Input: part model. Units: mm. Frame: model coordinates. Face numbers are marked on the shaded views. A direction names the side the tool comes from. Give positions to 0.01 mm unless a question says otherwise; leave off trailing zeros. Order: outer loops, then holes, each group sorted by start corner. A loop starts at its lowest first (then second) coordinate and runs counter-clockwise, first axis right, second up. Notation, with made-up numbers: (89, 17.25) - (110, 17.25) arc R31 ccw to (110, 42.25) - close; hole circle Ø6 at (46, -7). An arc over 180 degrees is marked (long way). Answer in a Markdown table with one row per item. Add a question column.
1. Ray query, line 1 (X direction, y = -9.5, z = -8); line 2 (Y direction, x = -27, z = -0.25); line 3 (Y direction, x = -21.5, z = -0.75). Return the intervals inside material, ascending. Write a range as [from, to].
2. Section query C-C on x = -14. Return loops of the section in (y, z).
3. Access query for the marked faces 1 and 2. Directions: +Z, -Z, +X, -X, +Y, -Y. A direction counts if a zero-diameter tool reaches every point of the face in a straight line with its end or side. Return the directions, or none.
4. Mould query, pull axis X, two halves, no side actions, for the marked faces 3, 4 and 5. Classes: released by +X, released by -X, zero draft, split by the parting line, or undercut.
5. Section query D-D on y = -22.5. Return loops of the section in (x, z).
6. Section query A-A on y = -14. Return loops of the section in (x, z).
7. Section query B-B on z = -0.5. Count the separate pieces of the cut face and the enclosed holes in it, and give its area (3 significant figures).
8. Contact query for flat-ended pins moving along their axis: pin 1 (1.2 mm diameter, centred on x = -14, y = -29, fed in from -Z); pin 2 (1.9 mm diameter, centred on x = -20, y = -2.5, fed in from -Z); pin 3 (0.5 mm diameter, centred on y = -29.5, z = -9, fed in from -X). Output: stop coordinate, or through.
```python
from build123d import *

# Parameters (mm, degrees)
SKETCH_2_W          = 31.092354585
SKETCH_2_H          = 31.600355601
EXTRUDE_1_DEPTH     = 1.5
SKETCH_3_R          = 1.9
SKETCH_3_R_2        = 0.85
EXTRUDE_2_DEPTH     = 2
SKETCH_4_W          = 31.092354585
SKETCH_4_H          = 31.600355601
SKETCH_4_R          = 0.9
SKETCH_4_R_2        = 0.95
EXTRUDE_3_DEPTH     = 13
CUT_EXTRUDE_1_REACH = 46.929
SKETCH_5_R          = 0.5
SKETCH_5_W          = 3.540807658
SKETCH_5_H          = 9.178364527
CUT_EXTRUDE_2_REACH = 46.95
SKETCH_6_W          = 4.41346869
SKETCH_6_H          = 8.209522231
CUT_EXTRUDE_3_REACH = 46.95
SKETCH_8_W          = 1
SKETCH_8_H          = 4
FILLET_1_R          = 1
FILLET_2_R          = 0.8


with BuildPart() as part:
    # 草图2 → 凸台-拉伸1 (new body)
    with BuildSketch(Plane.XY):
        with Locations((-13.658877318, -13.912877826)):
            Rectangle(SKETCH_2_W, SKETCH_2_H)
    extrude(amount=EXTRUDE_1_DEPTH)

    # 草图3 → 凸台-拉伸2 (add)
    # profile 1 of 2: a face of its own
    with BuildSketch(Plane(origin=(0, 0, 0), x_dir=(-1, 0, 0), z_dir=(0, 0, -1))):
        with Locations(Location((20.20004064, -2.16000508, 0), (0, 0, 180))):
            Circle(SKETCH_3_R)
        with Locations(Location((20.20004064, -2.16000508, 0), (0, 0, 180))):
            Circle(SKETCH_3_R_2, mode=Mode.SUBTRACT)
    # profile 2 of 2: a face of its own
    with BuildSketch(Plane(origin=(0, 0, 0), x_dir=(-1, 0, 0), z_dir=(0, 0, -1))):
        with Locations(Location((7.24001524, -25.6500508, 0), (0, 0, 180))):
            Circle(SKETCH_3_R)
        with Locations(Location((7.24001524, -25.6500508, 0), (0, 0, 180))):
            Circle(SKETCH_3_R_2, mode=Mode.SUBTRACT)
    extrude(amount=EXTRUDE_2_DEPTH)

    # 草图4 → 凸台-拉伸3 (add)
    # profile 1 of 2: a face of its own
    with BuildSketch(Plane(origin=(0, 0, 0), x_dir=(-1, 0, 0), z_dir=(0, 0, -1))):
        with Locations((13.658877318, -13.912877826)):
            Rectangle(SKETCH_4_W, SKETCH_4_H)
        Polygon((-0.387299975, -28.213055626), (-0.387299975, -23.216633759), (-0.387299975, 0.387299975), (22.708632743, 0.387299975), (27.70505461, 0.387299975), (27.70505461, -28.213055626), align=None, mode=Mode.SUBTRACT)
    # profile 2 of 2: a face of its own
    with BuildSketch(Plane(origin=(0, 0, 0), x_dir=(-1, 0, 0), z_dir=(0, 0, -1))):
        with BuildLine():
            Line((22.708632743, -28.200355601), (4.596421868, -28.200355601))
            ThreePointArc((4.596421868, -28.200355601), (3.261678652, -24.551376974), (-0.387299975, -23.216633759))
            Line((-0.387299975, -23.216633759), (-0.387299975, -28.213055626))
            Line((-0.387299975, -28.213055626), (27.70505461, -28.213055626))
            Line((27.70505461, -28.213055626), (27.70505461, 0.387299975))
            Line((27.70505461, 0.387299975), (22.708632743, 0.387299975))
            ThreePointArc((22.708632743, 0.387299975), (24.043375958, -3.261678652), (27.692354585, -4.596421868))
            Line((27.692354585, -4.596421868), (27.692354585, -23.216633759))
            ThreePointArc((27.692354585, -23.216633759), (24.043375958, -24.551376974), (22.708632743, -28.200355601))
        make_face()
        with Locations(Location((2.008877318, -25.812877826, 0), (0, 0, 180))):
            Circle(SKETCH_4_R, mode=Mode.SUBTRACT)
        with Locations(Location((25.308877318, -25.812877826, 0), (0, 0, 180))):
            Circle(SKETCH_4_R, mode=Mode.SUBTRACT)
        with Locations(Location((25.308877318, -2.012877826, 0), (0, 0, 180))):
            Circle(SKETCH_4_R_2, mode=Mode.SUBTRACT)
    extrude(amount=EXTRUDE_3_DEPTH)

    # 草图5 → 切除-拉伸1 (cut, up to next)
    with BuildSketch(Plane.ZY.offset(29.20505461), mode=Mode.PRIVATE) as cut_extrude_1_sk1:
        with Locations((-5.206157057, -6.409348234)):
            Circle(SKETCH_5_R)
    cut_extrude_1_tool1 = extrude(cut_extrude_1_sk1.sketch, amount=-CUT_EXTRUDE_1_REACH, mode=Mode.PRIVATE) & part.part
    # 草图5 → 切除-拉伸1 (cut, up to next)
    with BuildSketch(Plane.ZY.offset(29.20505461), mode=Mode.PRIVATE) as cut_extrude_1_sk2:
        with Locations((-5.206157057, -13.961165862)):
            Rectangle(SKETCH_5_W, SKETCH_5_H)
    cut_extrude_1_tool2 = extrude(cut_extrude_1_sk2.sketch, amount=-CUT_EXTRUDE_1_REACH, mode=Mode.PRIVATE) & part.part
    add(cut_extrude_1_tool1.solids().sort_by_distance((-29.205055, -6.409348, -5.206157))[0], mode=Mode.SUBTRACT)
    add(cut_extrude_1_tool2.solids().sort_by_distance((-29.205055, -13.961166, -5.206157))[0], mode=Mode.SUBTRACT)

    # 草图6 → 切除-拉伸2 (cut, up to next)
    with BuildSketch(Plane.XZ.offset(29.713055626), mode=Mode.PRIVATE) as cut_extrude_2_sk1:
        with Locations((-14.717018129, -8.895238884)):
            Rectangle(SKETCH_6_W, SKETCH_6_H)
    cut_extrude_2_tool1 = extrude(cut_extrude_2_sk1.sketch, amount=-CUT_EXTRUDE_2_REACH, mode=Mode.PRIVATE) & part.part
    add(cut_extrude_2_tool1.solids().sort_by_distance((-14.717018, -29.713056, -8.895239))[0], mode=Mode.SUBTRACT)

    # 草图8 → 切除-拉伸3 (cut, up to next)
    with BuildSketch(Plane(origin=(0, 1.887299975, 0), x_dir=(1, 0, 0), z_dir=(0, 1, 0)), mode=Mode.PRIVATE) as cut_extrude_3_sk1:
        with Locations((-7.644018288, 5.586156972)):
            Rectangle(SKETCH_8_W, SKETCH_8_H)
    cut_extrude_3_tool1 = extrude(cut_extrude_3_sk1.sketch, amount=-CUT_EXTRUDE_3_REACH, mode=Mode.PRIVATE) & part.part
    # 草图8 → 切除-拉伸3 (cut, up to next)
    with BuildSketch(Plane(origin=(0, 1.887299975, 0), x_dir=(1, 0, 0), z_dir=(0, 1, 0)), mode=Mode.PRIVATE) as cut_extrude_3_sk2:
        with Locations((-9.644018288, 5.586156972)):
            Rectangle(SKETCH_8_W, SKETCH_8_H)
    cut_extrude_3_tool2 = extrude(cut_extrude_3_sk2.sketch, amount=-CUT_EXTRUDE_3_REACH, mode=Mode.PRIVATE) & part.part
    # 草图8 → 切除-拉伸3 (cut, up to next)
    with BuildSketch(Plane(origin=(0, 1.887299975, 0), x_dir=(1, 0, 0), z_dir=(0, 1, 0)), mode=Mode.PRIVATE) as cut_extrude_3_sk3:
        with Locations((-5.644018288, 5.586156972)):
            Rectangle(SKETCH_8_W, SKETCH_8_H)
    cut_extrude_3_tool3 = extrude(cut_extrude_3_sk3.sketch, amount=-CUT_EXTRUDE_3_REACH, mode=Mode.PRIVATE) & part.part
    add(cut_extrude_3_tool1.solids().sort_by_distance((-7.644018, 1.8873, -5.586157))[0], mode=Mode.SUBTRACT)
    add(cut_extrude_3_tool2.solids().sort_by_distance((-9.644018, 1.8873, -5.586157))[0], mode=Mode.SUBTRACT)
    add(cut_extrude_3_tool3.solids().sort_by_distance((-5.644018, 1.8873, -5.586157))[0], mode=Mode.SUBTRACT)

    # 圆角1
    fillet_1_edges = [part.edges().sort_by_distance(p)[0] for p in [
        (-29.20505461, 1.887299975, -5.75),
        (1.887299975, 1.887299975, -5.75),
        (1.887299975, -29.713055626, -5.75),
        (-29.20505461, -29.713055626, -5.75),
    ]]
    fillet(fillet_1_edges, radius=FILLET_1_R)

    # 圆角2
    fillet_2_edges = [part.edges().sort_by_distance(p)[0] for p in [
        (-28.448704597, -9.371983599, -6.976560886),
        (-28.448704597, -9.371983599, -3.435753228),
        (-28.448704597, -18.550348126, -3.435753228),
        (-28.448704597, -18.550348126, -6.976560886),
    ]]
    fillet(fillet_2_edges, radius=FILLET_2_R)


solid = part.part
```
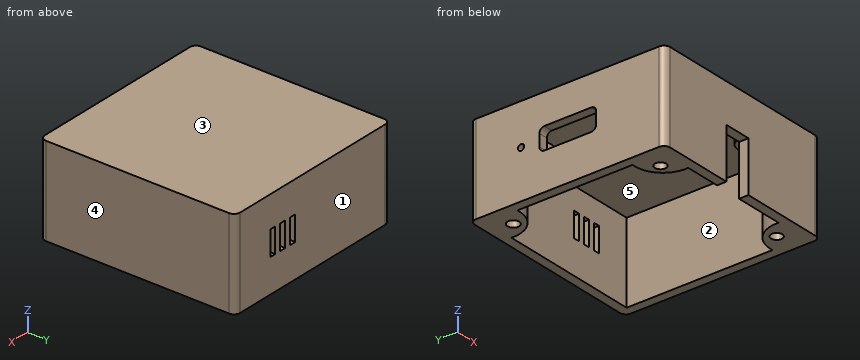
Answer:
| question | item | result |
|---|---|---|
| 1 | line 1 | x = [-29.21, -27.69], [0.39, 1.89] |
| 1 | line 2 | y = [-29.71, -23.21], [-4.6, 1.89] |
| 1 | line 3 | y = [-29.71, -28.2], [-3.55, -0.77], [0.39, 1.89] |
| 2 | outline | (-29.71, -4.79) - (-28.2, -4.79) - (-28.2, 0) - (0.39, 0) - (0.39, -13) - (1.89, -13) - (1.89, 1.5) - (-29.71, 1.5) - close |
| 3 | face 1 | +Z, -Z, +X, -X, +Y |
| 3 | face 2 | -Z |
| 4 | face 3 | zero draft |
| 4 | face 4 | released by +X |
| 4 | face 5 | undercut |
| 5 | outline | (-29.21, -13) - (-27.69, -13) - (-27.69, 0) - (0.39, 0) - (0.39, -13) - (1.89, -13) - (1.89, 1.5) - (-29.21, 1.5) - close |
| 6 | outline | (-29.21, -13) - (-27.69, -13) - (-27.69, -6.98) - (-29.21, -6.98) - close; (-29.21, -3.44) - (-27.69, -3.44) - (-27.69, 0) - (0.39, 0) - (0.39, -13) - (1.89, -13) - (1.89, 1.5) - (-29.21, 1.5) - close |
| 7 | separate pieces | 3 |
| 7 | enclosed holes | 6 |
| 7 | area | 250 mm² |
| 8 | pin 1 | stops at z = -4.79 |
| 8 | pin 2 | stops at z = -2 |
| 8 | pin 3 | stops at x = -29.05 |
